from build123d import *

# Parameters (mm, degrees)
PAD001_DEPTH = 15


with BuildPart() as batteryhold001:
    # Sketch002 → Pad001 (new body)
    with BuildSketch(Plane.XZ):
        with BuildLine():
            Line((0, 77.5), (10.75, 77.5))
            Line((10.75, 77.5), (10.75, 74.23403))
            ThreePointArc((10.75, 74.23403), (3.593187, 69.178911), (0.45, 61))
            Line((0, 61), (0.45, 61))
            Line((0, 77.5), (0, 61))
        make_face()
    extrude(amount=PAD001_DEPTH)


with BuildPart() as batteryhold001_1:
    # Body001 placement: moved
    add(batteryhold001.part.moved(Location((0, 24, 0))))


with BuildPart() as part_mirroring003:
    # Part__Mirroring003: instance of batteryHold001
    add(batteryhold001_1.part.mirror(Plane(origin=(0, 0, 0), x_dir=(0, 1, 0), z_dir=(0, 0, 1))))


with BuildPart() as part_mirroring003_1:
    # Part__Mirroring003 placement: moved
    add(part_mirroring003.part.moved(Location((0, 0, 74.5))))


with BuildPart() as part_mirroring004:
    # Part__Mirroring004: instance of Part__Mirroring003
    add(part_mirroring003_1.part.mirror(Plane(origin=(0, 0, 0), x_dir=(0, -1, 0), z_dir=(1, 0, 0))))


with BuildPart() as part_mirroring004_1:
    # Part__Mirroring004 placement: moved
    add(part_mirroring004.part.moved(Location((78, 0, 0))))


solid = part_mirroring004_1.part
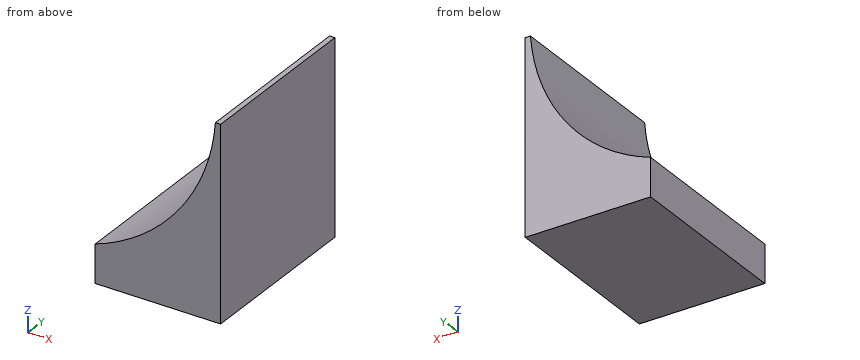
Geometry: final body of the model. Coordinates: model frame, mm. Give positions to 0.01 mm unless a question says otherwise; leave off trailing zeros. Loops run counter-clockwise (first coordinate to the right, second up) from the corner with the lowest first, then second, coordinate; pieces in that order, holes last. Notation, with made-up numbers: M 37,78 L 53,78 A16 cw 53,106 Z; hole C -13.75,5.25 d11. An arc over 180 degrees is marked long. Put each result on its own line as item: value.
1) Cut plane B-B, the plane x = 69. Return the cut outline in (y, z), plus the area to 3 significant figures.
Computed values:
outline: M 9,-3 L 24,-3 L 24,0.97 L 9,0.97 Z
area: 59.6 mm^2
2) Cut plane A-A, the plane y = 20.25. Return the cut outline in (x, z), plus the area to 3 significant figures.
Computed values:
outline: M 67.25,-3 L 78,-3 L 78,13.5 L 77.55,13.5 A15.1 cw 67.25,0.27 Z
area: 80.3 mm^2
3) Cut plane C-C, the plane z = 8.75. Return the cut outline in (x, y), plus the area to 3 significant figures.
Computed values:
outline: M 76.41,9 L 78,9 L 78,24 L 76.41,24 Z
area: 23.8 mm^2
4) First-contact query: P1, Ø6, axis at x = 70.5, y = 19, coming from the +Z side; P2, Ø2, axis at x = 71.5, y = 16, coming from the +Z side; P3, Ø5, axis at x = 72, z = 8.5, coming from the -Y side; P4, Ø2, axis at x = 69.5, y = 16, coming from the +Z side (3 decimals). Flat tips, straight axial feed; report the tip coordinate or a pass-through.
Computed values:
P1: stops at z = 4.26
P2: stops at z = 3.29
P3: passes through
P4: stops at z = 1.795
5) Material intervals for L1, parallel to Z at x = 72.5, y = 20.5; L2, parallel to X at y = 18.75, z = 11; L3, parallel to Z at x = 72.75, y = 22, sorted ascending. Write a range as from..to.
Computed values:
L1: z = -3..3.29
L2: x = 77.16..78
L3: z = -3..3.52
